The model under review builds one solid part; all positions refer to its coordinate system, in mm. Face numbers are marked on the shaded views. A direction names the side the tool comes from. Round coordinates to 2 decimals unless told otherwise and drop trailing zeros. Loops run counter-clockwise (first coordinate to the right, second up) from the corner with the lowest first, then second, coordinate; pieces in that order, holes last. Notation, with made-up numbers: M -4,62.25 L 55,62.25 A14 cw 55,77.25 Z; hole C 31,-37.5 d11. An arc over 180 degrees is marked long. Use a Markdown table: item, result. Add a question column.
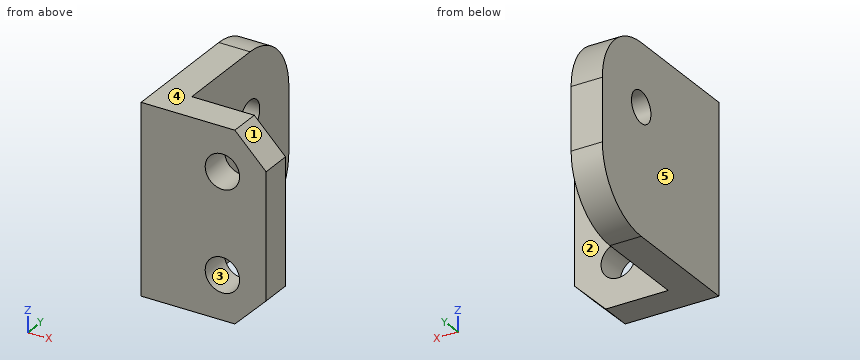
```python
from build123d import *

# Parameters (mm, degrees)
BOSS_EXTRUDE1_DEPTH        = 30
M6_TAPPED_HOLE2_D          = 5
F_5_5_5_5_DIAMETER_HOLE1_D = 5.5
CUT_EXTRUDE1_DEPTH         = 51.68530359
FILLET3_R                  = 10
CHAMFER1_SIZE              = 5


with BuildPart() as part:
    # Sketch1 → Boss-Extrude1 (new body)
    with BuildSketch(Plane.XY):
        Polygon((0, 0), (0, 38), (5, 38), (5, 5), (20, 5), (20, 0), align=None)
    extrude(amount=BOSS_EXTRUDE1_DEPTH)

    # M6 Tapped Hole2 (through all)
    with Locations(Plane(origin=(5, 0, 0), x_dir=(0, 0, -1), z_dir=(1, 0, 0))):
        with Locations((-20, 20)):
            Hole(M6_TAPPED_HOLE2_D / 2)

    # Ø5.5 (5.5) Diameter Hole1 (through all)
    with Locations(Plane(origin=(0, 5, 0), x_dir=(1, 0, 0), z_dir=(0, 1, 0))):
        with Locations((13, -7), (13, -23)):
            Hole(F_5_5_5_5_DIAMETER_HOLE1_D / 2)

    # Sketch13 → Cut-Extrude1 (cut, through all)
    with BuildSketch(Plane(origin=(5, 0, 0), x_dir=(0, 0, -1), z_dir=(1, 0, 0))):
        with BuildLine():
            Line((-20, 30), (0, 30))
            Line((0, 30), (0, 38))
            Line((0, 38), (-30, 38))
            Line((-30, 38), (-30, 20))
            ThreePointArc((-30, 20), (-27.071067812, 27.071067812), (-20, 30))
        make_face()
    extrude(amount=-CUT_EXTRUDE1_DEPTH, mode=Mode.SUBTRACT)

    # Fillet3
    fillet3_edges = [part.edges().sort_by_distance(p)[0] for p in [
        (2.5, 30, 0),
    ]]
    fillet(fillet3_edges, radius=FILLET3_R)

    # Chamfer1
    chamfer1_edges = [part.edges().sort_by_distance(p)[0] for p in [
        (20, 2.5, 0),
        (20, 2.5, 30),
    ]]
    chamfer(chamfer1_edges, length=CHAMFER1_SIZE)


solid = part.part
```
(1) Consider section C-C, the plane y = 2.25. Give the boundary of the cut face in (x, z), then the cut area to 3 significant figures.
(2) Consider section B-B, the plane x = 13. Give the boundary of the cut face in (y, z).
(3) Insertion check: pin 1 Ø5 at (x, z) = (6.5, 27) entering from +Y; pin 2 Ø7.5 at (x, z) = (9.5, 18) entering from +Y; pin 3 Ø10 at (y, z) = (18, 12.5) entering from +X. Each pin has a flat end and moves straight along its axis. Give the tip position at first contact, or say it passes through.
(4) For the marked faces 1 and 2, list the 3-axis set-ups (+Z, -Z, +X, -X, +Y, -Y) from which the entire face can be reached by the end or side of a thin tool; tool diameter is ignored.
(5) Draft analysis for pull direction Z (two halves, no side actions). For the marked faces 3, 4 and 5, state which applies: released by +Z, released by -Z, zero draft, split by the parting line, or undercut.
(6) Consider section A-A, the plane z = 18. Give the boundary of the cut face in (x, y), then the cut area to 3 significant figures.
(7) To check wall thickness, follow probe 1 along Z at (x, y) = (13, 4); probe 2 along Y at (x, z) = (2.05, 20); probe 3 along Y at (x, z) = (6.5, 3.5). State the ranges of each line that lie inside material, in increasing order.
(8) Consider section D-D, the plane y = 9.75. Give the boundary of the cut face in (x, z).
Found:
| question | item | result |
|---|---|---|
| 1 | outline | M 0,0 L 15,0 L 20,5 L 20,25 L 15,30 L 0,30 Z; hole C 13,7 d5.5; hole C 13,23 d5.5 |
| 1 | area | 527 mm^2 |
| 2 | outline | M 0,0 L 5,0 L 5,4.25 L 0,4.25 Z; M 0,9.75 L 5,9.75 L 5,20.25 L 0,20.25 Z; M 0,25.75 L 5,25.75 L 5,30 L 0,30 Z |
| 3 | pin 1 | stops at y = 28.66 |
| 3 | pin 2 | stops at y = 5 |
| 3 | pin 3 | stops at x = 5 |
| 4 | face 1 | +Z, +X, +Y, -Y |
| 4 | face 2 | +Z, -Z, +X, +Y |
| 5 | face 3 | undercut |
| 5 | face 4 | released by +Z |
| 5 | face 5 | zero draft |
| 6 | outline | M 0,0 L 20,0 L 20,5 L 5,5 L 5,18.5 L 0,18.5 Z; M 0,21.5 L 5,21.5 L 5,30 L 0,30 Z |
| 6 | area | 210 mm^2 |
| 7 | probe 1 | z = 0 to 4.25, 9.75 to 20.25, 25.75 to 30 |
| 7 | probe 2 | y = 0 to 17.5, 22.5 to 30 |
| 7 | probe 3 | y = 0 to 5 |
| 8 | outline | M 0,0 L 5,0 L 5,30 L 0,30 Z |
